The model under review builds one solid part; all positions refer to its coordinate system, in mm. A direction names the side the tool comes from. Give positions to 0.01 mm unless a question says otherwise; leave off trailing zeros. Loops run counter-clockwise (first coordinate to the right, second up) from the corner with the lowest first, then second, coordinate; pieces in that order, holes last. Notation, with made-up numbers: (58.25, -5) - (74.25, -5) arc R23 ccw to (74.25, 6) - close; hole circle Ø5 at (57, -25). An arc over 180 degrees is marked (long way). Return JSON: item names as keys, results as strings. Group by question number.
Autodesk Inventor part; units mm, degrees
ref_plane "YZ Plane" through (0, 0, 0) normal (1, 0, 0) x (0, 1, 0)
ref_plane "XZ Plane" through (0, 0, 0) normal (0, 1, 0) x (-1, 0, 0)
ref_plane "XY Plane" through (0, 0, 0) normal (0, 0, 1) x (1, 0, 0)
sketch "Sketch1" plane through (0, 0, 0) normal (0, 0, 1) x (1, 0, 0)
  line L0 (-4.5, 4.25) -> (4.25, 4.25)
  line L1 (4.25, 4.25) -> (4.25, -4.5)
  line L2 (4.25, -4.5) -> (-4.5, -4.5)
  line L3 (-4.5, -4.5) -> (-4.5, 4.25)
  point P0 (0, 0)
  dimension "d0" = 8.75
  dimension "d1" = 8.75
  dimension "d2" = 4.25
  dimension "d3" = 4.25
extrude "Extrusion1" add sketch "Sketch1" along normal blind 2.8
fillet "Fillet2" radius 1 3 edges at (4.25, 4.25, 1.4) (4.25, -0.125, 0) (-0.125, 4.25, 0)
sketch "Sketch10" plane through (0, 0, 2.8) normal (0, 0, 1) x (1, 0, 0)
  line L0 (4.25, 3.25) -> (4.25, -4.5)
  line L1 (-4.5, 4.25) -> (3.25, 4.25)
  line L2 (3.25, 3.25) -> (-17.75, 3.25)
  line L3 (-17.75, 3.25) -> (-17.75, -17.75)
  line L4 (-17.75, -17.75) -> (3.25, -17.75)
  line L5 (3.25, -17.75) -> (3.25, 3.25)
  point P0 (0, 0)
  dimension "d113" = 1
  dimension "d114" = 1
  dimension "d115" = 21
  dimension "d116" = 21
extrude "Extrusion8" add sketch "Sketch10" along normal blind 9
hole "Hole11" [suppressed]
sketch "Sketch11" plane through (0, 0, 2.8) normal (0, 0, -1) x (-1, 0, 0)
  line L0 (17.75, -17.75) -> (-3.25, -17.75)
  line L1 (17.75, 3.25) -> (17.75, -17.75)
  line L2 (4.5, 3.25) -> (17.75, 3.25)
  line L3 (12.25, 3.25) -> (17.75, 3.25)
  line L4 (17.75, 3.25) -> (17.75, -17.75)
  line L5 (17.75, -17.75) -> (-3.25, -17.75)
  line L6 (-3.25, -17.75) -> (-3.25, -10.75)
  line L7 (-3.25, -10.75) -> (2.25, -10.75)
  line L8 (2.25, -10.75) -> (12.25, -0.75)
  line L9 (12.25, -0.75) -> (12.25, 3.25)
  point P0 (0, 0)
  dimension "d146" = 14
  dimension "d158" = 4
  dimension "d254" = 15.5
  dimension "d255" = 45
extrude "Extrusion9" cut sketch "Sketch11" along normal through all both and the other way through all
hole "Hole12" [suppressed]
hole "Hole13" [suppressed]
chamfer "Chamfer3" [suppressed]
chamfer "Chamfer4" [suppressed]
sketch "Sketch18" plane through (0, 0, 0) normal (0, 0, -1) x (-1, 0, 0)
  line L0 (7, 5.953) -> (7, -1.75)
  line L1 (7, -1.75) -> (-6.3618, -1.75)
  line L2 (-3.25, 3.25) -> (4.5, 3.25)
  line L3 (-3.25, -4.5) -> (-3.25, 3.25)
  line L4 (7, 5.953) -> (-6.3618, 5.953)
  line L5 (-6.3618, 5.953) -> (-6.3618, -1.75)
  point P0 (0, 0)
  dimension "d226" = 2.703
  dimension "d227" = 3.1118
  dimension "d228" = 5
  dimension "d229" = 10.25
extrude "Extrusion12" cut sketch "Sketch18" against normal through all
hole "Hole16" at (-0.5, -1.75, 6.1) direction (0, -1, 0) diameter 1.1913 depth 4 tip angle 118
pattern_linear "Rectangular Pattern1" [suppressed]
chamfer "Chamfer7" [suppressed]
sketch "Sketch19" plane through (-4.5, -1.75, 0) normal (0, 1, 0) x (1, 0, 0)
  circle A0 centre (4, -6.1) radius 0.5956
  circle A1 centre (0.0078, -6.35) radius 0.5956
  point P0 (4.5, 0)
  dimension "d230" = 0.25
  dimension "d231" = 4
extrude "Extrusion13" cut sketch "Sketch19" against normal blind 4 contours A1
sketch "Sketch21" plane through (0, 0, 2.8) normal (0, 0, -1) x (-1, 0, 0)
  line L0 (7, 3.25) -> (7, -1.75)
  line L1 (7, -1.75) -> (4.5, -1.75)
  line L2 (-3.25, -10.75) -> (-3.25, -4.5)
  line L3 (-3.25, -10.75) -> (2.25, -10.75)
  line L4 (2.25, -10.75) -> (12.25, -0.75)
  line L5 (12.25, -0.75) -> (12.25, 3.25)
  line L6 (7, 3.25) -> (12.25, 3.25)
  line L7 (12.25, 4.25) -> (12.25, -0.75)
  line L8 (12.25, -0.75) -> (2.25, -10.75)
  line L9 (2.25, -10.75) -> (-4.25, -10.75)
  line L10 (-4.25, -10.75) -> (-4.25, -4.5)
  line L11 (-4.25, -4.5) -> (4.5, -4.5)
  line L12 (4.5, -4.5) -> (4.5, -1.75)
  line L13 (4.5, -1.75) -> (7, -1.75)
  line L14 (7, -1.75) -> (7, 4.25)
  line L15 (7, 4.25) -> (12.25, 4.25)
  line L16 (-3.25, -4.5) -> (4.5, -4.5)
  line L17 (4.5, -4.5) -> (4.5, -1.75)
  point P0 (0, 0)
  dimension "d236" = 1
  dimension "d237" = 1
extrude "Extrusion14" [suppressed]
chamfer "Chamfer8" [suppressed]
sketch "Sketch23" plane through (0, 0, 0) normal (0, 0, -1) x (-1, 0, 0)
  line L0 (-4.25, 4.25) -> (20.75, 4.25)
  line L1 (-4.25, -20.75) -> (-4.25, 4.25)
  line L2 (-1.875, -20.75) -> (-1.875, 1.875)
  line L3 (-1.875, 1.875) -> (20.75, 1.875)
  line L4 (4.5, -4.5) -> (4.5, -1.75)
  line L5 (20.75, 1.875) -> (20.75, 4.25)
  line L6 (-1.875, -20.75) -> (-4.25, -20.75)
  point P0 (0, 0)
  dimension "d245" = 2.375
  dimension "d249" = 1.875
  dimension "d250" = 1.875
  dimension "d251" = 25
  dimension "d252" = 25
extrude "Extrusion16" cut sketch "Sketch23" against normal through all
hole "Hole10" at (-9.768, 1.875, 7.317) direction (0, -1, 0) diameter 2.3876 depth 5 tip angle 118 countersink diameter 2.794 countersink angle 120
fillet "Fillet4" radius 1 2 edges at (-1.3125, -4.5, 0) (-4.5, -3.125, 0)
hole "Hole18" at (1.875, -7.75, 8.5) direction (-1, 0, 0) diameter 2.3876 depth 4.826 tip angle 118 countersink diameter 2.794 countersink angle 120
hole "Hole17" at (-0.9768, -7.795, 2.8) direction (0, 0, 1) diameter 2.3876 depth 3.9878 tip angle 118 countersink diameter 2.794 countersink angle 120
sketch "Sketch24" plane through (0, 0, 11.8) normal (0, 0, 1) x (1, 0, 0)
  line L0 (1.875, -10.75) -> (1.875, -1.75)
  line L1 (-7, 1.875) -> (1.875, 1.875)
  line L2 (1.875, 1.875) -> (1.875, -3.125)
  line L3 (1.875, -3.125) -> (-7, -3.125)
  line L4 (-7, 1.875) -> (-7, -3.125)
  line L5 (-7, 1.875) -> (-12.25, 1.875)
  point P0 (0, 0)
  dimension "d276" = 5
extrude "Extrusion17" cut sketch "Sketch24" against normal blind 4
sketch "Sketch25" plane through (0, 0, 11.8) normal (0, 0, 1) x (1, 0, 0)
  line L0 (-12.25, 1.875) -> (-12.25, -0.75)
  line L1 (-12.25, -0.75) -> (-2.25, -10.75)
  line L2 (-12.25, 1.875) -> (-6.5, 1.875)
  line L3 (-6.5, 1.875) -> (-6.5, -6.5)
  line L4 (-6.5, -6.5) -> (-12.25, -6.5)
  line L5 (-12.25, -6.5) -> (-12.25, 1.875)
  point P0 (0, 0)
extrude "Extrusion18" cut sketch "Sketch25" against normal blind 2 contours L2 L3 L1 L0
sketch "Sketch26" plane through (0, 0, 11.8) normal (0, 0, 1) x (1, 0, 0)
  line L0 (-6.5, -3.125) -> (-6.5, -6.5)
  line L1 (-6.5, -6.5) -> (-2.25, -10.75)
  line L2 (-2.25, -10.75) -> (1.875, -10.75)
  line L3 (1.875, -10.75) -> (1.875, -3.125)
  line L4 (-6.5, -3.125) -> (-1.125, -3.125)
  line L5 (-1.125, -3.125) -> (-1.125, -10.75)
  line L6 (-1.125, -10.75) -> (-6.5, -10.75)
  line L7 (-6.5, -10.75) -> (-6.5, -3.125)
  point P0 (0, 0)
  dimension "d281" = 3
extrude "Extrusion19" cut sketch "Sketch26" against normal up to surface (2 mm away) contours L4 L5 L2 L1 L0
fillet "Fillet5" radius 1.3 1 edges at (-7, -3.125, 8.8)
properties part number "FOX-ME-121-05" material "Aluminum-6061"
1) Draft analysis for pull direction Y (two halves, no side actions). For faces 5 (the face through (-10, 1.875, 5)), 6 (the face through (-1, -3, 0)), 7 (the face through (-1.335, -6.656, 4.88)), 8 (the face through (-1.357, -4.199, 0.285)), state which applies: +Y half, -Y half, draft (parallel to the pull), parting line (faces both ways), or undercut.
2) Tool access review of faces 1 (the face through (-1, -4.5, 2)), 2 (the face through (-4.965, -3.722, 6.712)), 3 (the face through (-0.63, -8.76, 7.86)), 4 (the face through (-6.609, -2.754, 8.786)): name each direction out of +Z, -Z, +X, -X, +Y, -Y from which nothing blocks a thin tool from reaching the whole face with its end or side.
3) We need section A-A, the plane y = -5.5. Write out the cut boundary in (x, z) (3 decimals), plus the area to 3 significant figures.
4) We need section B-B, the plane z = 6.35. Count the separate pieces of the cut face and the enclosed holes in it, plus the area to 3 significant figures.
5) For pin 1 Ø3 at (y, z) = (-1.5, 7.5) entering from +X (3 decimals); pin 2 Ø1 at (x, z) = (-9, 7.5) entering from +Y; pin 3 Ø2 at (y, z) = (-8, 11) entering from -X (3 decimals); pin 4 Ø1.2 at (x, z) = (-3.5, 9.5) entering from +Y (3 decimals), all flat-tipped, find the tip position at first contact; note any pin that passes through.
6) To check wall thickness, follow line 1 (Z direction, x = -0.5, y = -3); line 2 (Y direction, x = -1.8, z = 8.5) (3 decimals); line 3 (Z direction, x = 0.45, y = -7.75). State the ranges of each line that lie inside material, in increasing order.
Findings:
{
 "1": {"face 5": "+Y half", "face 6": "draft", "face 7": "undercut", "face 8": "-Y half"},
 "2": {"face 1": "-Z, +X, -X, -Y", "face 2": "+Y", "face 3": "+X", "face 4": "+Z, +X, +Y"},
 "3": {"outline": "(-7.5, 2.8) - (1.875, 2.8) - (1.875, 11.8) - (-1.125, 11.8) - (-1.125, 9.8) - (-7.5, 9.8) - close; hole circle Ø1.191 at (-4.492, 6.35); hole circle Ø1.191 at (-0.5, 6.1)", "area": "69.4 mm^2"},
 "4": {"separate pieces": "2", "enclosed holes": "1", "area": "75.5 mm^2"},
 "5": {"pin 1": "stops at x = 1.875", "pin 2": "stops at y = 1.81", "pin 3": "stops at x = -1.125", "pin 4": "stops at y = -3.125"},
 "6": {"line 1": "z = 0 to 5.5, 6.7 to 7.8", "line 2": "y = -10.75 to -8.944, -6.556 to -3.125", "line 3": "z = 2.8 to 7.31, 9.69 to 11.8"}
}
